Here's how the part is built. I have some questions about the finished solid (model axes, mm). A direction names the side the tool comes from. Give positions to 0.01 mm unless a question says otherwise; leave off trailing zeros. Loops run counter-clockwise (first coordinate to the right, second up) from the corner with the lowest first, then second, coordinate; pieces in that order, holes last. Notation, with made-up numbers: M -9.75,63.5 L 45.25,63.5 A31 ccw 45.25,87.5 Z; hole C 66.5,19 d7. An arc over 180 degrees is marked long. Answer as CSV lines item,"result". Start each with the question number.
Item 1: If we mould it in two halves opening along Y, with no side actions, what happens to faces 4 (the flat face through (91, -19.05, 0)), 5 (the flat face through (-11, 306, 9.525)), 6 (the flat face through (345, 0, 0))? For each: released by +Y, released by -Y, zero draft, split by the parting line, or undercut.
Item 2: Will this pin go through, and if not, where does the flat tip stop? P1, Ø1.6, axis at x = 196.85, z = 5.4, coming from the -Y side.
Item 3: I want a section at A-A on x = 54. List the corners of the cut face in (y, z) for me (3 decimals).
Item 4: I want a section at B-B on y = 73. List the corners of the cut face in (x, z) for me (3 decimals), plus the area to 3 significant figures.
Item 5: For faces 1 (the flat face through (103, 0, 0)), 2 (the flat face through (-11, 306, -9.525)), 3 (the flat face through (228.6, -9, 0)), which set-ups out of +Z, -Z, +X, -X, +Y, -Y let a thin tool reach every point of the face, with its end or its side?
Item 6: If I drill on line 1 along Z through (x, y) = (196.85, -4.75) (3 decimals); line 2 along X through (y, z) = (76.5, 7); line 3 along Y through (x, z) = (260, 5.75), over which ranges is the centre line in solid material (lowest first)? Write a range as from..to.
from build123d import *

# Parameters (mm, degrees)
F1_DEPTH = 9.525
F2_R     = 1.35255
F3_DEPTH = 19.051


with BuildPart() as f1:
    # F0 (on Top) → F1 (new body, symmetric)
    with BuildSketch(Plane.XY):
        Polygon((457.2, 609.6), (457.2, 0), (228.6, 0), (228.6, -19.05), (476.25, -19.05), (476.25, 628.65), (-19.05, 628.65), (-19.05, -19.05), (203.2, -19.05), (203.2, 0), (0, 0), (0, 609.6), align=None)
    extrude(amount=F1_DEPTH, both=True)

    # F2 (on face) → F3 (cut, through all)
    with BuildSketch(Plane(origin=(0, 0, 0), x_dir=(-1, 0, 0), z_dir=(0, 1, 0))):
        with Locations((-247.65, 5.3975)):
            Circle(F2_R)
        with Locations((-247.65, -5.3975)):
            Circle(F2_R)
        with Locations((-234.95, 5.3975)):
            Circle(F2_R)
        with Locations((-234.95, -5.3975)):
            Circle(F2_R)
        with Locations((-196.85, 5.3975)):
            Circle(F2_R)
        with Locations((-184.15, 5.3975)):
            Circle(F2_R)
        with Locations((-184.15, -5.3975)):
            Circle(F2_R)
        with Locations((-196.85, -5.3975)):
            Circle(F2_R)
    extrude(amount=-F3_DEPTH, mode=Mode.SUBTRACT)


solid = f1.part
Result:
1,face 4,"released by -Y"
1,face 5,"zero draft"
1,face 6,"undercut"
2,P1,"y = 609.6"
3,outline,"M -19.05,-9.525 L 0,-9.525 L 0,9.525 L -19.05,9.525 Z; M 609.6,-9.525 L 628.65,-9.525 L 628.65,9.525 L 609.6,9.525 Z"
4,outline,"M -19.05,-9.525 L 0,-9.525 L 0,9.525 L -19.05,9.525 Z; M 457.2,-9.525 L 476.25,-9.525 L 476.25,9.525 L 457.2,9.525 Z"
4,area,"726 mm^2"
5,face 1,"+Z, -Z"
5,face 2,"-Z, +X, -X, +Y, -Y"
5,face 3,"+Z, -Z, -Y"
6,line 1,"-9.525..-6.75, -4.045..4.045, 6.75..9.525"
6,line 2,"-19.05..0, 457.2..476.25"
6,line 3,"-19.05..0, 609.6..628.65"
